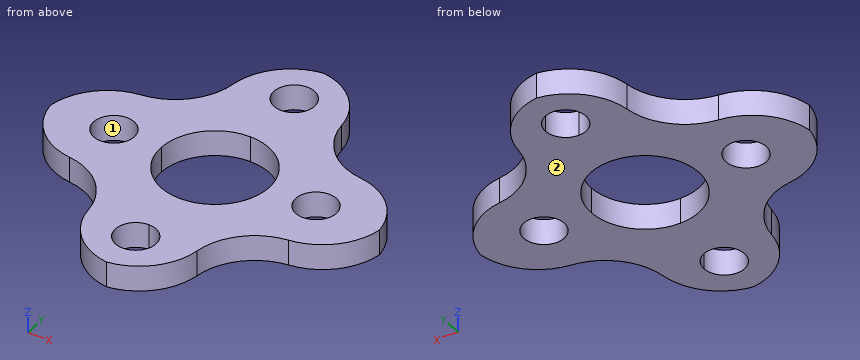
from build123d import *

# Parameters (mm, degrees)
F1_R        = 13.1
F1_R_2      = 1.6
F2_DEPTH    = 2
F3_R        = 5
F4_DEPTH    = 25
F5_T1_DEPTH = 33.3713058975


# Not quite as in the source:
# - a fillet or chamfer that OpenCascade refuses, or shapes differently, is made with other operations: its cross-section is extruded or revolved along the edge and cut away or added


with BuildPart() as f2:
    # F1 (on Top) → F2 (new body)
    with BuildSketch(Plane.XY):
        Circle(F1_R)
        with BuildLine():
            ThreePointArc((1.6, -9.5), (-1.1313708499, -10.6313708499), (0, -7.9))
            ThreePointArc((0, -7.9), (1.1313708499, -8.3686291501), (1.6, -9.5))
        make_face(mode=Mode.SUBTRACT)
        with Locations((-8, 0)):
            Circle(F1_R_2, mode=Mode.SUBTRACT)
        with BuildLine():
            ThreePointArc((-4.25, 0), (-3.00520382, 3.00520382), (0, 4.25))
            ThreePointArc((0, 4.25), (3.00520382, 3.00520382), (4.25, 0))
            ThreePointArc((4.25, 0), (3.00520382, -3.00520382), (0, -4.25))
            ThreePointArc((0, -4.25), (-3.00520382, -3.00520382), (-4.25, 0))
        make_face(mode=Mode.SUBTRACT)
        with BuildLine():
            ThreePointArc((9.6, 0), (8, -1.6), (6.4, 0))
            ThreePointArc((6.4, 0), (8, 1.6), (9.6, 0))
        make_face(mode=Mode.SUBTRACT)
        with BuildLine():
            ThreePointArc((1.6, 9.5), (1.1313708499, 8.3686291501), (0, 7.9))
            ThreePointArc((0, 7.9), (-1.1313708499, 10.6313708499), (1.6, 9.5))
        make_face(mode=Mode.SUBTRACT)
    extrude(amount=F2_DEPTH)

    # F3 (on face) → F4 (cut)
    with BuildSketch(Plane.XY.offset(2)):
        with Locations((-9.2630988335, 9.2630988335)):
            Circle(F3_R)
        with Locations((9.2630988335, -9.2630988335)):
            Circle(F3_R)
        with Locations((-9.2630988335, -9.2630988335)):
            Circle(F3_R)
        with Locations((9.2630988335, 9.2630988335)):
            Circle(F3_R)
    extrude(amount=-F4_DEPTH, mode=Mode.SUBTRACT)

    # F5: fillet of radius 5 on 8 edges, made by hand

    # F5_s2 → F5_t1 (cut)
    with BuildSketch(Plane.XY.offset(-15.6856529487)):
        with BuildLine():
            ThreePointArc((1.0767599787, 13.0556726348), (-2.4959833234, 11.9459923629), (-4.298657973, 8.667845155))
            ThreePointArc((-4.298657973, 8.667845155), (-4.4028928152, 10.437150561), (-5.1178235319, 12.0589337131))
            ThreePointArc((-5.1178235319, 12.0589337131), (-2.0810864422, 12.9336413751), (1.0767599787, 13.0556726348))
        make_face()
        with BuildLine():
            ThreePointArc((-8.667845155, 4.298657973), (-11.9459923629, 2.4959833234), (-13.0556726348, -1.0767599787))
            ThreePointArc((-13.0556726348, -1.0767599787), (-12.9336413751, 2.0810864422), (-12.0589337131, 5.1178235319))
            ThreePointArc((-12.0589337131, 5.1178235319), (-10.437150561, 4.4028928152), (-8.667845155, 4.298657973))
        make_face()
        with BuildLine():
            ThreePointArc((13.0556726348, -1.0767599787), (11.9459923629, 2.4959833234), (8.667845155, 4.298657973))
            ThreePointArc((8.667845155, 4.298657973), (10.437150561, 4.4028928152), (12.0589337131, 5.1178235319))
            ThreePointArc((12.0589337131, 5.1178235319), (12.9336413751, 2.0810864422), (13.0556726348, -1.0767599787))
        make_face()
        with BuildLine():
            ThreePointArc((4.298657973, 8.667845155), (2.4959833234, 11.9459923629), (-1.0767599787, 13.0556726348))
            ThreePointArc((-1.0767599787, 13.0556726348), (2.0810864422, 12.9336413751), (5.1178235319, 12.0589337131))
            ThreePointArc((5.1178235319, 12.0589337131), (4.4028928152, 10.437150561), (4.298657973, 8.667845155))
        make_face()
        with BuildLine():
            ThreePointArc((13.0556726348, 1.0767599787), (11.9459923629, -2.4959833234), (8.667845155, -4.298657973))
            ThreePointArc((8.667845155, -4.298657973), (10.437150561, -4.4028928152), (12.0589337131, -5.1178235319))
            ThreePointArc((12.0589337131, -5.1178235319), (12.9336413751, -2.0810864422), (13.0556726348, 1.0767599787))
        make_face()
        with BuildLine():
            ThreePointArc((-1.0767599787, -13.0556726348), (2.4959833234, -11.9459923629), (4.298657973, -8.667845155))
            ThreePointArc((4.298657973, -8.667845155), (4.4028928152, -10.437150561), (5.1178235319, -12.0589337131))
            ThreePointArc((5.1178235319, -12.0589337131), (2.0810864422, -12.9336413751), (-1.0767599787, -13.0556726348))
        make_face()
        with BuildLine():
            ThreePointArc((-13.0556726348, 1.0767599787), (-11.9459923629, -2.4959833234), (-8.667845155, -4.298657973))
            ThreePointArc((-8.667845155, -4.298657973), (-10.437150561, -4.4028928152), (-12.0589337131, -5.1178235319))
            ThreePointArc((-12.0589337131, -5.1178235319), (-12.9336413751, -2.0810864422), (-13.0556726348, 1.0767599787))
        make_face()
        with BuildLine():
            ThreePointArc((-4.298657973, -8.667845155), (-2.4959833234, -11.9459923629), (1.0767599787, -13.0556726348))
            ThreePointArc((1.0767599787, -13.0556726348), (-2.0810864422, -12.9336413751), (-5.1178235319, -12.0589337131))
            ThreePointArc((-5.1178235319, -12.0589337131), (-4.4028928152, -10.437150561), (-4.298657973, -8.667845155))
        make_face()
    extrude(amount=F5_T1_DEPTH, mode=Mode.SUBTRACT)


solid = f2.part
The listing builds one solid part. Answer for the finished solid, in the listing's coordinates (mm). Face numbers are marked on the shaded views. Coordinates: 2 decimals unless noted, no trailing zeros. Write each loop counter-clockwise with the first axis right and the second up, starting at its lowest first coordinate (ties: lowest second). Pieces come first, ordered by that corner, then holes. Notation, with made-up numbers: (2.25, 78) -> (11.25, 78) arc R22 cw to (11.25, 86) -> close; hole circle Ø5 at (76.5, 70). An arc over 180 degrees is marked (long way). One line per question, with ' | ' between items.
1. Straight lines are drawn through the part: line 1 (X direction, y = -9.5, z = 0.55); line 2 (Y direction, x = -0.5, z = 1.1); line 3 (Y direction, x = -2, z = 0.1). For each, find the intervals that lie inside material, in ascending order.
Verdict:
line 1: x = -4.13 to -1.6, 1.6 to 4.13 | line 2: y = -12.93 to -11.02, -7.98 to -4.22, 4.22 to 7.98, 11.02 to 12.93 | line 3: y = -12.3 to -3.75, 3.75 to 12.3
2. Section C-C (x = 8.25) is taken. Determine the outline of the cut face in (y, z).
Verdict:
outline: (-4.37, 0) -> (-1.58, 0) -> (-1.58, 2) -> (-4.37, 2) -> close; (1.58, 0) -> (4.37, 0) -> (4.37, 2) -> (1.58, 2) -> close
3. Section D-D (y = 6.75) is taken. Determine the outline of the cut face in (x, z), and give its area (3 significant figures).
Verdict:
outline: (-4.94, 0) -> (4.94, 0) -> (4.94, 2) -> (-4.94, 2) -> close | area: 19.8 mm^2
4. Section A-A (z = 0.55) is taken. Determine the outline of the cut face in (x, y).
Verdict:
outline: (-13.03, 0) arc R5 ccw to (-8.67, -4.3) arc R5 cw to (-4.3, -8.67) arc R5 ccw to (0, -13.03) arc R5 ccw to (4.3, -8.67) arc R5 cw to (8.67, -4.3) arc R5 ccw to (13.03, 0) arc R5 ccw to (8.67, 4.3) arc R5 cw to (4.3, 8.67) arc R5 ccw to (0, 13.03) arc R5 ccw to (-4.3, 8.67) arc R5 cw to (-8.67, 4.3) arc R5 ccw to start; hole circle Ø3.2 at (-8, 0); hole circle Ø8.5 at (0, 0); hole circle Ø3.2 at (0, -9.5); hole circle Ø3.2 at (0, 9.5); hole circle Ø3.2 at (8, 0)
5. Given pin 1 Ø4 at (x, y) = (-8, 0) entering from -Z, flat-ended and moving along its own axis, determine where the tip first touches the part or whether it passes through.
Verdict:
pin 1: stops at z = 0
6. Section B-B (y = -3.75) is taken. Determine the outline of the cut face in (x, z), and give its area (3 significant figures).
Verdict:
outline: (-10.42, 0) -> (-2, 0) -> (-2, 2) -> (-10.42, 2) -> close; (2, 0) -> (10.42, 0) -> (10.42, 2) -> (2, 2) -> close | area: 33.7 mm^2
7. For a pull along X with two mould halves and no side action, classify the marked faces 1 and 2 as released by +X, released by -X, zero draft, split by the parting line, or undercut.
Verdict:
face 1: undercut | face 2: zero draft
